Geometry check sheet. Reference: the model listing, model coordinates, mm. A direction names the side the tool comes from. Coordinates: 2 decimals unless noted, no trailing zeros. Write each loop counter-clockwise with the first axis right and the second up, starting at its lowest first coordinate (ties: lowest second). Pieces come first, ordered by that corner, then holes. Notation, with made-up numbers: (1.25, 78) -> (45.25, 78) arc R23 ccw to (45.25, 103) -> close; hole circle Ø3 at (66.25, 34.25). An arc over 180 degrees is marked (long way). Answer in a Markdown table with one row per item. Add a question column.
Q1. Section check B-B, the plane x = 16.5. Record the boundary of the cut face in (y, z).
Q2. Gauge pin test, flat ends, axial feed: P1, Ø12, axis at x = -7, y = -5, coming from the -Z side; P2, Ø1.5, axis at y = -2.5, z = 4, coming from the +X side. Record the tip position at first contact, or that the pin passes through.
Q3. Tool access check on faces 1 (the face through (11.568, -23.066, 4.93)), 2 (the face through (19.93, -17.605, 4.93)). Record the directions out of +Z, -Z, +X, -X, +Y, -Y that give a thin tool (end or side, any length) a straight path to the whole face; none if there is none.
Q4. Thickness scan on line 1 (Y direction, x = 22, z = 2.5); line 2 (Y direction, x = -18, z = 5); line 3 (X direction, y = 7, z = 9.25). Record the ranges inside material, lowest first.
Q5. Section check C-C, the plane y = -5. Record the boundary of the cut face in (x, z), and give its area (3 significant figures).
Q6. Release check for a two-part mould opening along X. For faces 3 (the face through (22.15, 21.99, 4.93)), 4 (the face through (7.444, -20.638, 4.93)), 5 (the face through (-5, 25, 5)), 6 (the face through (-25, -7, 5)) record: pulls with the +X half, pulls with the -X half, needs draft (parallel to the pull), parting line crosses it, or undercut.
Q7. Section check A-A, the plane z = 1.25. Record the boundary of the cut face in (x, y).
```python
from build123d import *

# Parameters (mm, degrees)
F1_DEPTH = 10


with BuildPart() as f1:
    # F0 (on Top) → F1 (new body)
    with BuildSketch(Plane.XY):
        with BuildLine():
            ThreePointArc((25, 15), (22.071068, 22.071068), (15, 25))
            Line((15, 25), (-25, 25))
            Line((-25, 25), (-25, 10))
            ThreePointArc((-25, 10), (-20, 5), (-25, 0))
            Line((-25, 0), (-25, -15))
            ThreePointArc((-25, -15), (-22.071068, -22.071068), (-15, -25))
            Line((-15, -25), (0, -25))
            ThreePointArc((0, -25), (2.080642, -20.94077), (6.590941, -20.259862))
            ThreePointArc((6.590941, -20.259862), (7.455256, -20.644347), (8.231687, -21.184741))
            Line((8.231687, -21.184741), (15, -25))
            Line((15, -25), (25, -10))
            ThreePointArc((25, -10), (20, -5), (25, 0))
            Line((25, 0), (25, 15))
        make_face()
    extrude(amount=F1_DEPTH)


solid = f1.part
```
Calculated:
| question | item | result |
|---|---|---|
| 1 | outline | (-22.75, 0) -> (24.89, 0) -> (24.89, 10) -> (-22.75, 10) -> close |
| 2 | P1 | stops at z = 0 |
| 2 | P2 | stops at x = 21.2 |
| 3 | face 1 | +Z, -Z, -Y |
| 3 | face 2 | +Z, -Z, +X, -Y |
| 4 | line 1 | y = -14.5 to -9, -1 to 22.14 |
| 4 | line 2 | y = -24.54 to 25 |
| 4 | line 3 | x = -20.42 to 25 |
| 5 | outline | (-25, 0) -> (20, 0) -> (20, 10) -> (-25, 10) -> close |
| 5 | area | 450 mm² |
| 6 | face 3 | pulls with the +X half |
| 6 | face 4 | undercut |
| 6 | face 5 | needs draft |
| 6 | face 6 | pulls with the -X half |
| 7 | outline | (-25, -15) arc R10 ccw to (-15, -25) -> (0, -25) arc R5 cw to (6.59, -20.26) arc R5 cw to (8.23, -21.18) -> (15, -25) -> (25, -10) arc R5 cw to (25, 0) -> (25, 15) arc R10 ccw to (15, 25) -> (-25, 25) -> (-25, 10) arc R5 cw to (-25, 0) -> close |
